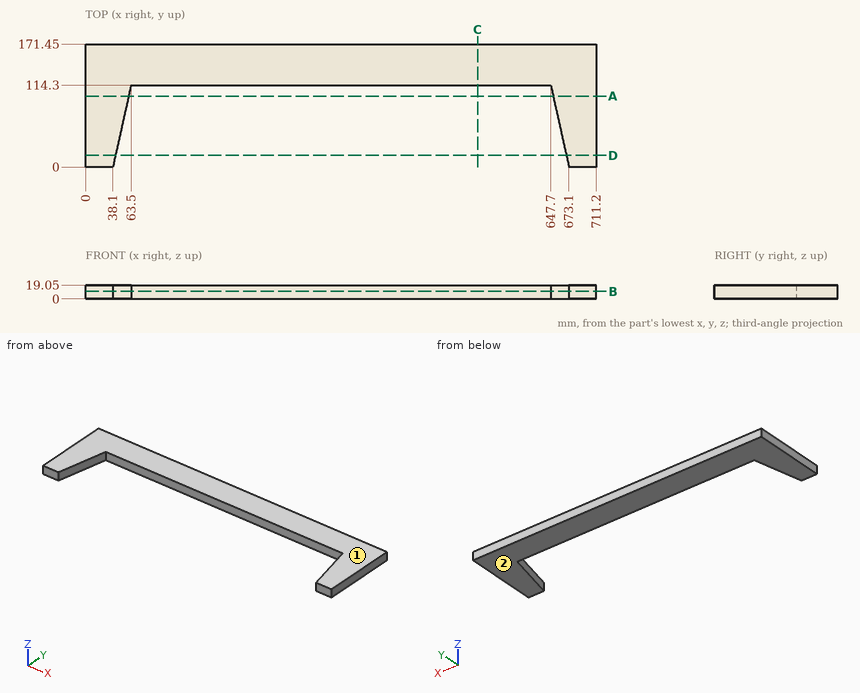
Geometry: see drawing. Coordinates: mm, zero at the bounding-box minimum. Give positions to 0.01 mm unless a question says otherwise; leave off trailing zeros. Order: outer loops, then holes, each group sorted by start corner. A loop starts at its lowest first (then second) coordinate and runs counter-clockwise, first axis right, second up. Notation, with made-up numbers: M 75,73 L 128,73 A37 cw 128,111 Z; hole C -13,-23 d3. An arc over 180 degrees is marked long. Answer as a JSON object with one key per item and string values.
1. Ray query, line 1 (Y direction, x = 562, z = 16.5); line 2 (X direction, y = 20, z = 13.5); line 3 (X direction, y = 61, z = 15.5). Return the intervals inside material, ascending. Write a range as [from, to].
Result sheet:
{"line 1": "[114.3, 171.45]", "line 2": "[0, 42.54], [668.66, 711.2]", "line 3": "[0, 51.66], [659.54, 711.2]"}
2. Cut plane C-C, the plane x = 546. Output: boundary loops of the cut face in (y, z), and give its area (3 significant figures).
Result sheet:
{"outline": "M 114.3,0 L 171.45,0 L 171.45,19.05 L 114.3,19.05 Z", "area": "1,090 mm²"}
3. Cut plane D-D, the plane y = 16.5. Output: boundary loops of the cut face in (x, z).
Result sheet:
{"outline": "M 0,0 L 41.77,0 L 41.77,19.05 L 0,19.05 Z; M 669.43,0 L 711.2,0 L 711.2,19.05 L 669.43,19.05 Z"}
4. Cut plane A-A, the plane y = 99. Output: boundary loops of the cut face in (x, z).
Result sheet:
{"outline": "M 0,0 L 60.1,0 L 60.1,19.05 L 0,19.05 Z; M 651.1,0 L 711.2,0 L 711.2,19.05 L 651.1,19.05 Z"}
5. Cut plane B-B, the plane z = 10.25. Output: boundary loops of the cut face in (x, y).
Result sheet:
{"outline": "M 0,0 L 38.1,0 L 63.5,114.3 L 647.7,114.3 L 673.1,0 L 711.2,0 L 711.2,171.45 L 0,171.45 Z"}
6. First-contact query: P1, Ø1.5, axis at x = 484.5, z = 12.5, coming from the -Y side. Flat tip, straight axial feed; report the tip coordinate or a pass-through.
Result sheet:
{"P1": "y = 114.3"}
7. Pull-direction query (Z, two-part tool) for the marked faces 1 and 2; classes: +Z half, -Z half, draft (parallel to the pull), parting line (faces both ways), or undercut.
Result sheet:
{"face 1": "+Z half", "face 2": "-Z half"}
